Geometry check sheet. Reference: the model listing, model coordinates, mm. Face numbers are marked on the shaded views. A direction names the side the tool comes from. Round coordinates to 2 decimals unless told otherwise and drop trailing zeros. Loops run counter-clockwise (first coordinate to the right, second up) from the corner with the lowest first, then second, coordinate; pieces in that order, holes last. Notation, with made-up numbers: M 18.25,85 L 48.25,85 A30 cw 48.25,124 Z; hole C 7.25,39 d3. An arc over 180 degrees is marked long. Use one line per item in the form item = value. Start each with the question number.
1. Set-up check for the marked faces 5 and 6: record each of +Z, -Z, +X, -X, +Y, -Y from which the full face is reachable in a straight line by a thin tool's end or side.
2. Cross-section at A-A (x = 0). Record the boundary of the cut face in (y, z), then the cut area to 3 significant figures.
3. Draft check along X on the marked faces 1, 2, 3 and 4. Enter one of: pulls with the +X half, pulls with the -X half, needs draft (parallel to the pull), parting line crosses it, or undercut.
4. Material ranges on line 1 (Z direction, x = 13.5, y = 0); line 2 (Y direction, x = 6, z = 23.75); line 3 (Y direction, x = 11.25, z = 12.5), recorded low to high.
5. Cross-section at C-C (y = 11.5). Record the boundary of the cut face in (x, z).
6. Go/stop test with flat-tipped pins: pin 1 (2.5 mm diameter, centred on x = 0.5, z = 18, fed in from +Y); pin 2 (4 mm diameter, centred on x = 9, z = 5, fed in from +Y); pin 3 (2.5 mm diameter, centred on y = 0, z = 12.5, fed in from +X); pin 4 (10 mm diameter, centred on x = 3.5, y = 3.5, fed in from +Z). Record where each tip stops, or that it passes through.
7. Cross-section at B-B (z = 10). Record the boundary of the cut face in (x, y), then the cut area to 3 significant figures.
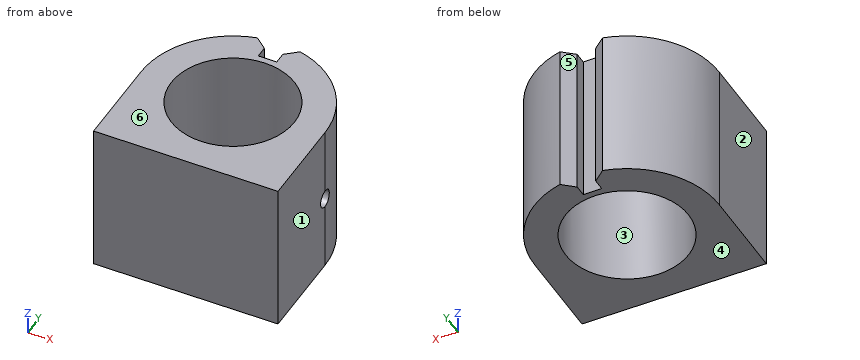
Autodesk Inventor part; units mm, degrees
ref_plane "YZ Plane" through (0, 0, 0) normal (1, 0, 0) x (0, 1, 0)
ref_plane "XZ Plane" through (0, 0, 0) normal (0, 1, 0) x (-1, 0, 0)
ref_plane "XY Plane" through (0, 0, 0) normal (0, 0, 1) x (1, 0, 0)
sketch "Skizze3" plane through (0, 0, 0) normal (0, 0, 1) x (1, 0, 0)
  circle A0 centre (0, 0) radius 10
  arc A1 (15, 0) -> (-15, 0) centre (0, 0) ccw
  line L0 (15, 0) -> (15, -15)
  line L1 (15, -15) -> (-15, -15)
  line L2 (-15, -15) -> (-15, 0)
  line L3 (-15, 15) -> (15, -15) construction
  line L4 (15, 15) -> (-15, -15) construction
extrude "Extrusion2" add sketch "Skizze3" along normal blind 25
sketch "Skizze4" plane through (0, 0, 25) normal (0, 0, 1) x (1, 0, 0)
  circle A0 centre (0, 0) radius 10 construction
  line L0 (15, -15) -> (15, 0) construction
  arc A1 (15, 0) -> (-15, 0) centre (0, 0) ccw construction
  line L1 (-15, 0) -> (-15, -15) construction
  line L2 (-15, -15) -> (15, -15) construction
  line L3 (-1.5, 19) -> (1.5, 19)
  line L4 (1.5, 19) -> (1.5, 11)
  line L5 (1.5, 11) -> (-1.5, 11)
  line L6 (-1.5, 11) -> (-1.5, 19)
  arc A2 (15, 0) -> (-15, 0) centre (0, 0) ccw
  line L7 (-1.5, 19) -> (1.5, 11) construction
  line L8 (1.5, 19) -> (-1.5, 11) construction
  point P0 (0, 15)
  dimension "d9" = 3
  dimension "d10" = 8
extrude "Extrusion3" cut sketch "Skizze4" against normal through all
chamfer "Fase1" distance 2 angle 45 2 edges at (-1.5, 14.9248, 12.5) (1.5, 14.9248, 12.5)
sketch "Skizze5" plane through (15, -15, 0) normal (1, 0, 0) x (0, 0, -1)
  line L0 (0, 15) -> (-25, 15)
  circle A0 centre (-12.5, 15) radius 1.45
  dimension "d16" = 2.9
extrude "Extrusion4" cut sketch "Skizze5" against normal blind 6
properties part number "pipe_ruler"
Reported:
q1.face_5 = +Z, -Z, +Y
q1.face_6 = +Z, +X, -X, +Y, -Y
q2.outline = M -15,0 L -10,0 L -10,25 L -15,25 Z; M 10,0 L 11,0 L 11,25 L 10,25 Z
q2.area = 150 mm²
q3.face_1 = pulls with the +X half
q3.face_2 = pulls with the -X half
q3.face_3 = undercut
q3.face_4 = needs draft
q4.line_1 = 0 to 11.05, 13.95 to 25
q4.line_2 = -15 to -8, 8 to 13.75
q4.line_3 = -15 to -1.45, 1.45 to 9.92
q5.outline = M -9.63,0 L -1.5,0 L -1.5,25 L -9.63,25 Z; M 1.5,0 L 9.63,0 L 9.63,25 L 1.5,25 Z
q6.pin_1 = 13.14
q6.pin_2 = 13.27
q6.pin_3 = -9.92
q6.pin_4 = through
q7.outline = M -15,-15 L 15,-15 L 15,0 A15 ccw 3.47,14.59 L 1.5,12.92 L 1.5,11 L -1.5,11 L -1.5,12.92 L -3.47,14.59 A15 ccw -15,0 Z; hole C 0,0 d20
q7.area = 473 mm²
